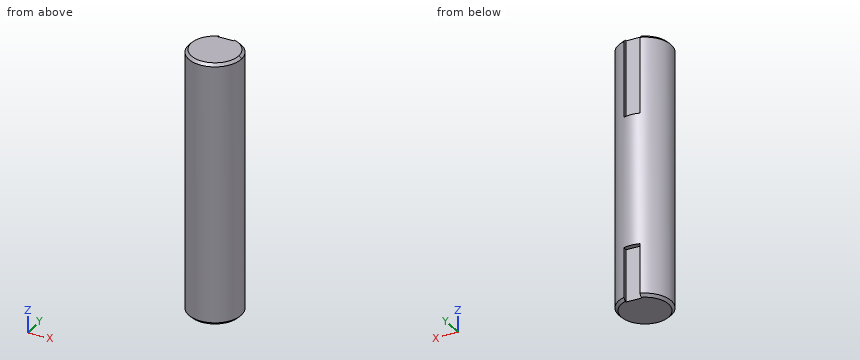
from build123d import *

# Parameters (mm, degrees)
SKETCH1_R           = 10
BOSS_EXTRUDE1_DEPTH = 100
SKETCH2_W           = 6
SKETCH2_H           = 2.85006478
CUT_EXTRUDE1_DEPTH  = 30
SKETCH3_W           = 6
SKETCH3_H           = 2.660897005
CUT_EXTRUDE2_DEPTH  = 20
CHAMFER1_SIZE       = 1


with BuildPart() as part:
    # Sketch1 → Boss-Extrude1 (new body)
    with BuildSketch(Plane.XY):
        Circle(SKETCH1_R)
    extrude(amount=BOSS_EXTRUDE1_DEPTH)

    # Sketch2 → Cut-Extrude1 (cut)
    with BuildSketch(Plane.XY.offset(100)):
        with Locations((0, 9.42503239)):
            Rectangle(SKETCH2_W, SKETCH2_H)
    extrude(amount=-CUT_EXTRUDE1_DEPTH, mode=Mode.SUBTRACT)

    # Sketch3 → Cut-Extrude2 (cut)
    with BuildSketch(Plane(origin=(0, 0, 0), x_dir=(-1, 0, 0), z_dir=(0, 0, -1))):
        with Locations((0, 9.330448503)):
            Rectangle(SKETCH3_W, SKETCH3_H)
    extrude(amount=-CUT_EXTRUDE2_DEPTH, mode=Mode.SUBTRACT)

    # Chamfer1
    chamfer1_edges = [part.edges().sort_by_distance(p)[0] for p in [
        (-5.916079783, -8.062257748, 0),
        (-5.916079783, -8.062257748, 100),
    ]]
    chamfer(chamfer1_edges, length=CHAMFER1_SIZE)


solid = part.part
Could you check a few things on this model? Use its own coordinates, in mm. Give positions to 0.01 mm unless a question says otherwise; leave off trailing zeros. Loops run counter-clockwise (first coordinate to the right, second up) from the corner with the lowest first, then second, coordinate; pieces in that order, holes last. Notation, with made-up numbers: (83, 77.5) -> (90, 77.5) arc R37 ccw to (90, 113.5) -> close; hole circle Ø3 at (83, 48.25). An arc over 180 degrees is marked (long way). Answer as CSV lines item,"result". Start each with the question number.
(1) I need wall thicknesses on probe 1 along X at (y, z) = (0.5, 44); probe 2 along Z at (x, y) = (9, -0.25); probe 3 along X at (y, z) = (3.75, 32). Which ranges of each line are inside material? Lowest first, please.
(2) I'm going to push flat-ended pins straight in: pin 1 Ø1.7 at (y, z) = (9, 14) entering from +X; pin 2 Ø0.8 at (y, z) = (9, 85) entering from -X; pin 3 Ø5 at (x, z) = (1, 14.5) entering from +Y. Where does each tip first touch, or does it pass through?
(3) If we section it at C-C on z = 67.5: Write out the boundary of the cut face in (x, y).
(4) If we section it at B-B on z = 10: Write out the boundary of the cut face in (x, y), then the cut area to 3 significant figures.
(5) If we section it at A-A on x = 0: Write out the boundary of the cut face in (y, z), then the cut area to 3 significant figures.
Computed:
1,probe 1,"x = -9.99 to 9.99"
1,probe 2,"z = 0 to 100"
1,probe 3,"x = -9.27 to 9.27"
2,pin 1,"stops at x = 5.79"
2,pin 2,"stops at x = -5.1"
2,pin 3,"stops at y = 9.54"
3,outline,"circle Ø20 at (0, 0)"
4,outline,"(-3, 8) -> (-3, 9.54) arc R10 ccw (long way) to (3, 9.54) -> (3, 8) -> close"
4,area,"303 mm2"
5,outline,"(-10, 1) -> (-9, 0) -> (8, 0) -> (8, 20) -> (10, 20) -> (10, 70) -> (8, 70) -> (8, 100) -> (-9, 100) -> (-10, 99) -> close"
5,area,"1,900 mm2"
